Part model, mm, in its own coordinate system. A direction names the side the tool comes from. Round coordinates to 2 decimals unless told otherwise and drop trailing zeros. Loops run counter-clockwise (first coordinate to the right, second up) from the corner with the lowest first, then second, coordinate; pieces in that order, holes last. Notation, with made-up numbers: M 2,-23.75 L 23,-23.75 A26 ccw 23,-5.75 Z; hole C 65.5,-24.5 d1. An arc over 180 degrees is marked long. Put each result on its own line as item: value. Start each with the question number.
Autodesk Inventor part; units mm, degrees
ref_plane "YZ Plane" through (0, 0, 0) normal (1, 0, 0) x (0, 1, 0)
ref_plane "XZ Plane" through (0, 0, 0) normal (0, 1, 0) x (-1, 0, 0)
ref_plane "XY Plane" through (0, 0, 0) normal (0, 0, 1) x (1, 0, 0)
sketch "Sketch1" plane through (0, 0, 0) normal (0, 0, 1) x (1, 0, 0)
  line L0 (0, 0) -> (-16, 0)
  line L1 (-16, 0) -> (-8, 13.8564)
  line L2 (-8, 13.8564) -> (0, 0)
  line L3 (0, 0) -> (-16, 0)
  line L4 (-8, 15.8564) -> (-17.7321, -1)
  line L5 (-17.7321, -1) -> (1.7321, -1)
  line L6 (1.7321, -1) -> (-8, 15.8564)
  dimension "d4" = 16
  dimension "d5" = 1
extrude "Extrusion1" add sketch "Sketch1" along normal blind 5
properties part number "dishRing_3DPrint"
1. Cut at B-B, the plane z = 2.5. Give the cut face in (x, y), and give its area (3 significant figures).
2. Cut at A-A, the plane x = -3. Give the cut face in (y, z), and give its area (3 significant figures).
3. Cut at C-C, the plane y = 12.5. Give the cut face in (x, z).
4. Drop a flat-ended pin along its axis: pin 1 (1.5 mm diameter, centred on y = 7.5, z = 1, fed in from +X). Give the stop position or say it passes through.
5. Wall check: L1, parallel to Y at x = -13, z = 4.2; L2, parallel to Y at x = -12, z = 1.5; L3, parallel to X at y = 12.25, z = 3.2. Give the ranges that are in metal, low to high.
6. Which spindle directions (+Z, -Z, +X, -X, +Y, -Y) get a long thin tool onto all of the face, cutting with end or side? Do faces 5 (the flat face through (-4.06, 7.03, 2.46)), 6 (the flat face through (-12.798, 7.546, 2.465)). Say none if no direction does.
7. Mould opens along Y. For faces 1 (the flat face through (-8.8, -0.6, 0)), 2 (the flat face through (-8, 0, 2)), 3 (the flat face through (-3.066, 7.31, 2.465)), 4 (the flat face through (-12.056, 6.831, 2.465)) say: released by +Y, released by -Y, zero draft, split by the parting line, or undercut.
Results list:
1. outline: M -17.73,-1 L 1.73,-1 L -8,15.86 Z; hole M -16,0 L 0,0 L -8,13.86 Z
1. area: 53.2 mm^2
2. outline: M -1,0 L 0,0 L 0,5 L -1,5 Z; M 5.2,0 L 7.2,0 L 7.2,5 L 5.2,5 Z
2. area: 15.0 mm^2
3. outline: M -9.94,0 L -8.78,0 L -8.78,5 L -9.94,5 Z; M -7.22,0 L -6.06,0 L -6.06,5 L -7.22,5 Z
4. pin 1: stops at x = -2.74
5. L1: y = -1 to 0, 5.2 to 7.2
5. L2: y = -1 to 0, 6.93 to 8.93
5. L3: x = -10.08 to -8.93, -7.07 to -5.92
6. face 5: +Z, -Z
6. face 6: +Z, -Z, -X, +Y
7. face 1: zero draft
7. face 2: undercut
7. face 3: released by +Y
7. face 4: undercut
